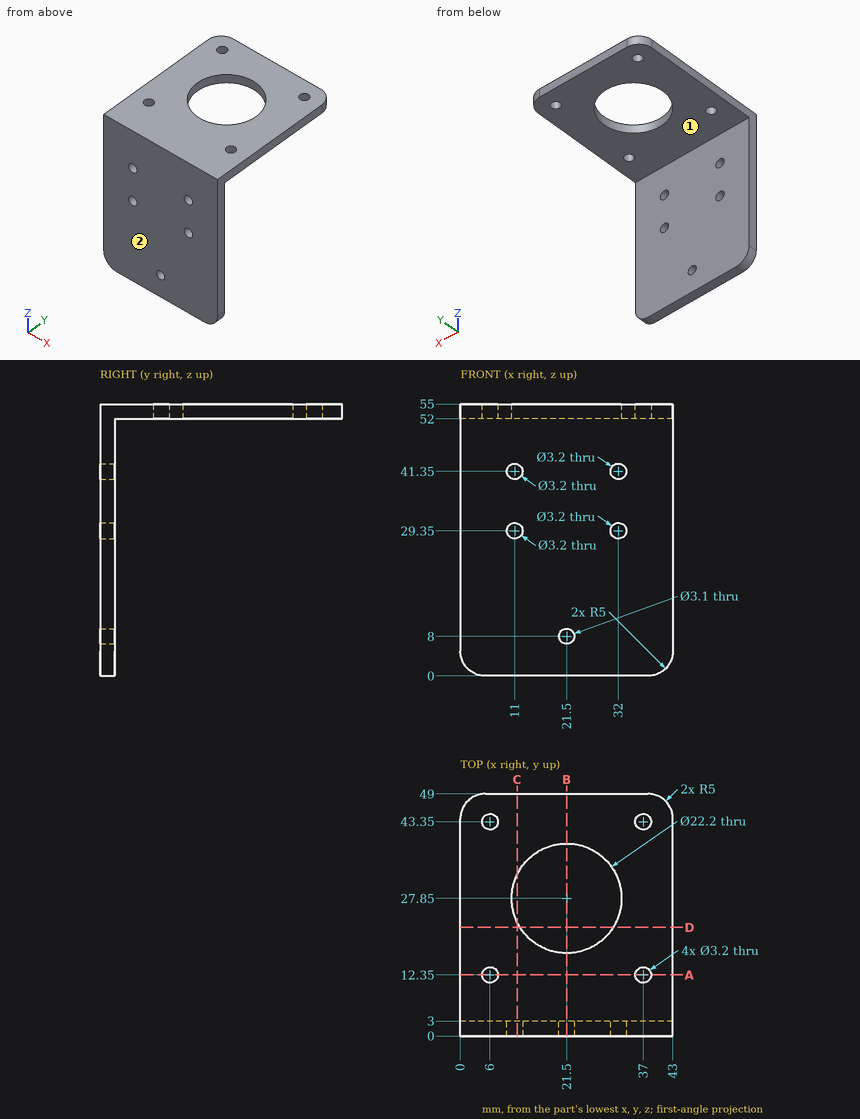
Design review of the part shown in the three views and the two pictorial views. Dimensions are in mm from the part's minimum x, y and z. A direction names the side the tool comes from. Give positions to 0.01 mm unless a question says otherwise; leave off trailing zeros. Write each loop counter-clockwise with the first axis right and the second up, starting at its lowest first coordinate (ties: lowest second). Pieces come first, ordered by that corner, then holes.
Item 1: Insertion check: P1, Ø21.5, axis at x = 22, y = 24.5, coming from the -Z side; P2, Ø3, axis at x = 6, y = 43.35, coming from the +Z side; P3, Ø4, axis at x = 11, z = 29.35, coming from the +Y side. Each pin has a flat end and moves straight along its axis. Give the tip position at first contact, or say it passes through.
Item 2: Take a section at B-B (x = 21.5). Give the boundary of the cut face in (y, z).
Item 3: Wall thickness on probe 1 along Y at (x, z) = (6, 54); probe 2 along X at (y, z) = (1.4, 41.35); probe 3 along Z at (x, y) = (32, 2): over which ranges is each line inside the solid? List them lowest first.
Item 4: Take a section at D-D (y = 22). Give the boundary of the cut face in (x, z), and give its area (3 significant figures).
Item 5: Machinability: for the marked faces 1 and 2, which of the approach directions +Z, -Z, +X, -X, +Y, -Y give a long, thin tool a straight path to every point of the face, cutting with its end or side? Answer none if there is none.
Item 6: Take a section at A-A (y = 12.35). Give the boundary of the cut face in (x, z), and give its area (3 significant figures).
Item 7: Take a section at C-C (x = 11.5). Give the boundary of the cut face in (y, z), and give its area (3 significant figures).
Established:
1. P1: stops at z = 52
1. P2: passes through
1. P3: stops at y = 3
2. outline: (0, 0) - (3, 0) - (3, 6.45) - (0, 6.45) - close; (0, 9.55) - (3, 9.55) - (3, 52) - (16.75, 52) - (16.75, 55) - (0, 55) - close; (38.95, 52) - (49, 52) - (49, 55) - (38.95, 55) - close
3. probe 1: y = 0 to 10.75, 13.95 to 41.75, 44.95 to 49
3. probe 2: x = 0 to 9.4, 12.6 to 30.4, 33.6 to 43
3. probe 3: z = 0 to 27.75, 30.95 to 39.75, 42.95 to 55
4. outline: (0, 52) - (12.07, 52) - (12.07, 55) - (0, 55) - close; (30.93, 52) - (43, 52) - (43, 55) - (30.93, 55) - close
4. area: 72.4 mm2
5. face 1: -Z, +X, -X, +Y
5. face 2: +Z, -Z, +X, -X, -Y
6. outline: (0, 52) - (4.4, 52) - (4.4, 55) - (0, 55) - close; (7.6, 52) - (35.4, 52) - (35.4, 55) - (7.6, 55) - close; (38.6, 52) - (43, 52) - (43, 55) - (38.6, 55) - close
6. area: 110 mm2
7. outline: (0, 0) - (3, 0) - (3, 27.83) - (0, 27.83) - close; (0, 30.87) - (3, 30.87) - (3, 39.83) - (0, 39.83) - close; (0, 42.87) - (3, 42.87) - (3, 52) - (23.03, 52) - (23.03, 55) - (0, 55) - close; (32.67, 52) - (49, 52) - (49, 55) - (32.67, 55) - close
7. area: 256 mm2
